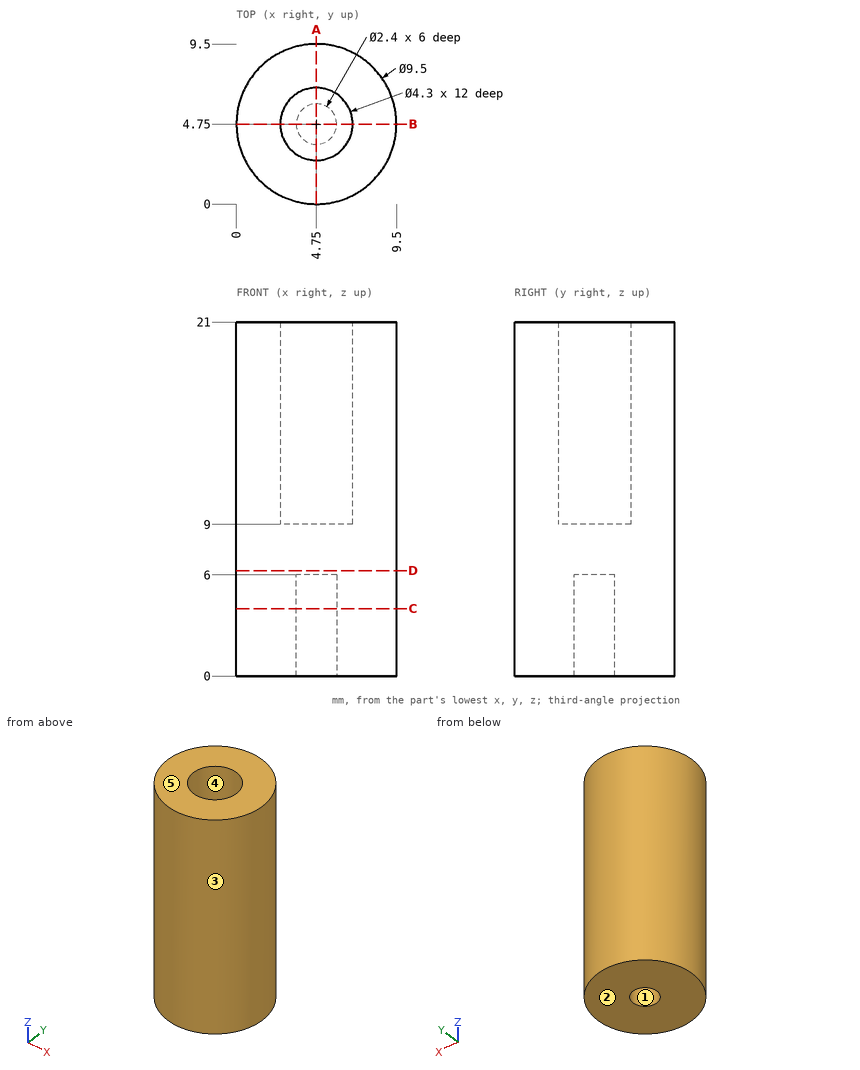
Geometry: see drawing. Coordinates: mm, zero at the bounding-box minimum. A direction names the side the tool comes from. Round coordinates to 2 decimals unless told otherwise and drop trailing zeros. Loops run counter-clockwise (first coordinate to the right, second up) from the corner with the lowest first, then second, coordinate; pieces in that order, holes last. Notation, with made-up numbers: (34.5, 24.25) -> (79.5, 24.25) arc R27 ccw to (79.5, 43.25) -> close; hole circle Ø3 at (15.25, 9). An arc over 180 degrees is marked (long way). Use one line per item in the form item = value. Start each with the question number.
Item 1: Contact query for flat-ended pins moving along their axis: pin 1 Ø0.7 at (x, y) = (5, 5) entering from -Z; pin 2 Ø1.5 at (y, z) = (3, 9.5) entering from +X; pin 3 Ø5 at (x, z) = (2, 8) entering from +Y. Output: stop coordinate, or through.
Item 2: Set-up query: the marked faces 1 and 2. Return all of +Z, -Z, +X, -X, +Y, -Y with unobstructed straight access to the full face (end or side cutting, diameter ignored); none if empty.
Item 3: Section query D-D on z = 6.25. Return the cut outline in (x, y), then the cut area to 3 significant figures.
Item 4: Mould query, pull axis Y, two halves, no side actions, for the marked faces 3, 4 and 5. Classes: pulls with the +Y half, pulls with the -Y half, needs draft (parallel to the pull), parting line crosses it, or undercut.
Item 5: Material intervals for L1, parallel to Y at x = 4.75, z = 13; L2, parallel to Y at x = 3, z = 18.25; L3, parallel to Z at x = 5.25, y = 6.5, sorted ascending. Write a range as from..to.
Item 6: Section query A-A on x = 4.75. Return the cut outline in (y, z).
Item 7: Section query C-C on z = 4. Return the cut outline in (x, y).
Ans:
q1.pin_1 = 6
q1.pin_2 = 9.39
q1.pin_3 = 9.49
q2.face_1 = -Z
q2.face_2 = -Z, +X, -X, +Y, -Y
q3.outline = circle Ø9.5 at (4.75, 4.75)
q3.area = 70.9 mm^2
q4.face_3 = parting line crosses it
q4.face_4 = undercut
q4.face_5 = needs draft
q5.L1 = 0..2.6, 6.9..9.5
q5.L2 = 0.33..3.5, 6..9.17
q5.L3 = 0..9
q6.outline = (0, 0) -> (3.55, 0) -> (3.55, 6) -> (5.95, 6) -> (5.95, 0) -> (9.5, 0) -> (9.5, 21) -> (6.9, 21) -> (6.9, 9) -> (2.6, 9) -> (2.6, 21) -> (0, 21) -> close
q7.outline = circle Ø9.5 at (4.75, 4.75); hole circle Ø2.4 at (4.75, 4.75)
